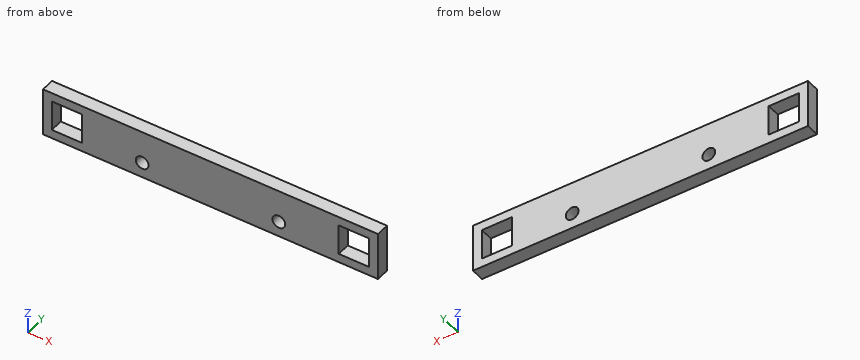
```python
from build123d import *

# Parameters (mm, degrees)
ESQUISSE1_W        = 76
ESQUISSE1_H        = 10.9
ESQUISSE1_R        = 1.45
ESQUISSE1_W_2      = 6.9
ESQUISSE1_H_2      = 6.9
BOSS_EXTRU_1_DEPTH = 3


with BuildPart() as part:
    # Esquisse1 → Boss.-Extru.1 (new body)
    with BuildSketch(Plane(origin=(0, 0, 0), x_dir=(1, 0, 0), z_dir=(0, 1, 0))):
        with Locations((38, 5.45)):
            Rectangle(ESQUISSE1_W, ESQUISSE1_H)
        with Locations(Location((22.5, 7.4, 0), (0, 0, 270))):
            Circle(ESQUISSE1_R, mode=Mode.SUBTRACT)
        with Locations(Location((53.5, 7.4, 0), (0, 0, 270))):
            Circle(ESQUISSE1_R, mode=Mode.SUBTRACT)
        with Locations((5.45, 5.45)):
            Rectangle(ESQUISSE1_W_2, ESQUISSE1_H_2, mode=Mode.SUBTRACT)
        with Locations((70.55, 5.45)):
            Rectangle(ESQUISSE1_W_2, ESQUISSE1_H_2, mode=Mode.SUBTRACT)
    extrude(amount=BOSS_EXTRU_1_DEPTH)


solid = part.part
```
CAD build for the part. Positions are in the model's coordinates, mm. Round coordinates to 2 decimals unless told otherwise and drop trailing zeros. Write each loop counter-clockwise with the first axis right and the second up, starting at its lowest first coordinate (ties: lowest second). Pieces come first, ordered by that corner, then holes. Notation, with made-up numbers: (45.5, -26) - (80.5, -26) arc R32 cw to (80.5, 4) - close; hole circle Ø6 at (-10, -8). An arc over 180 degrees is marked (long way). Write item = value, one per line. Start each with the question number.
Q1. Band-saw the part on C-C (x = 22.5). Give the cut face in (y, z), then the cut area to 3 significant figures.
Q2. Band-saw the part on A-A (z = -7.4). Give the cut face in (x, y), then the cut area to 3 significant figures.
Q3. Band-saw the part on B-B (y = 2.35). Give the cut face in (x, z).
Q4. Probe L1, parallel to X at y = 1.8, z = -7.4; L2, parallel to X at y = 0.4, z = -3.25; L3, parallel to Z at x = 6.5, y = 1.85. List the from-to ranges inside material, lowest first. Write a range as from..to.
Q5. Band-saw the part on D-D (z = -3.5). Give the cut face in (x, y).
Answers below:
q1.outline = (0, -10.9) - (3, -10.9) - (3, -8.85) - (0, -8.85) - close; (0, -5.95) - (3, -5.95) - (3, 0) - (0, 0) - close
q1.area = 24.0 mm2
q2.outline = (0, 0) - (2, 0) - (2, 3) - (0, 3) - close; (8.9, 0) - (21.05, 0) - (21.05, 3) - (8.9, 3) - close; (23.95, 0) - (52.05, 0) - (52.05, 3) - (23.95, 3) - close; (54.95, 0) - (67.1, 0) - (67.1, 3) - (54.95, 3) - close; (74, 0) - (76, 0) - (76, 3) - (74, 3) - close
q2.area = 169 mm2
q3.outline = (0, -10.9) - (76, -10.9) - (76, 0) - (0, 0) - close; hole (2, -8.9) - (8.9, -8.9) - (8.9, -2) - (2, -2) - close; hole circle Ø2.9 at (22.5, -7.4); hole circle Ø2.9 at (53.5, -7.4); hole (67.1, -8.9) - (74, -8.9) - (74, -2) - (67.1, -2) - close
q4.L1 = 0..2, 8.9..21.05, 23.95..52.05, 54.95..67.1, 74..76
q4.L2 = 0..2, 8.9..67.1, 74..76
q4.L3 = -10.9..-8.9, -2..0
q5.outline = (0, 0) - (2, 0) - (2, 3) - (0, 3) - close; (8.9, 0) - (67.1, 0) - (67.1, 3) - (8.9, 3) - close; (74, 0) - (76, 0) - (76, 3) - (74, 3) - close
